```python
from build123d import *

# Parameters (mm, degrees)
BOSS_EXTRUDE1_DEPTH = 6
SKETCH2_W           = 0.8
SKETCH2_H           = 5.9
CUT_EXTRUDE1_DEPTH  = 0.5
SKETCH3_R           = 0.2
BOSS_EXTRUDE2_DEPTH = 2.5


with BuildPart() as part:
    # Sketch1 → Boss-Extrude1 (new body)
    with BuildSketch(Plane(origin=(0, 0, 0), x_dir=(0, 0, -1), z_dir=(1, 0, 0))):
        Polygon((-7.5, -6.8), (-7.5, 3.2), (-2.5, 3.2), (-2.5, -4.8), (2.5, -4.8), (2.5, 3.2), (7.5, 3.2), (7.5, -6.8), align=None)
    extrude(amount=BOSS_EXTRUDE1_DEPTH)

    # Sketch2 → Cut-Extrude1 (cut)
    with BuildSketch(Plane(origin=(0, 0, -7.5), x_dir=(-1, 0, 0), z_dir=(0, 0, -1))):
        with Locations((-3, 0.25)):
            Rectangle(SKETCH2_W, SKETCH2_H)
    cut_extrude1 = extrude(amount=-CUT_EXTRUDE1_DEPTH, mode=Mode.SUBTRACT)

    # Mirror1: Cut-Extrude1 across plane
    add(cut_extrude1.mirror(Plane.XY), mode=Mode.SUBTRACT)

    # Sketch3 → Boss-Extrude2 (add)
    with BuildSketch(Plane.XZ.offset(6.8)):
        with Locations((1.73, -5)):
            Circle(SKETCH3_R)
        with Locations((4.27, -5)):
            Circle(SKETCH3_R)
        with Locations((4.27, 5)):
            Circle(SKETCH3_R)
        with Locations((1.73, 5)):
            Circle(SKETCH3_R)
    extrude(amount=BOSS_EXTRUDE2_DEPTH)


solid = part.part
```
The listing builds one solid part. Answer for the finished solid, in the listing's coordinates (mm). A direction names the side the tool comes from. Round coordinates to 2 decimals unless told otherwise and drop trailing zeros. Loops run counter-clockwise (first coordinate to the right, second up) from the corner with the lowest first, then second, coordinate; pieces in that order, holes last.
Q1. Section D-D, the plane x = 1.73 is taken. Determine the outline of the cut face in (y, z).
Q2. Which of the six approach directions +Z, -Z, +X, -X, +Y, -Y give full straight-line access (tool end or side, diameter ignored) to faces 1 (the face through (3, 3.2, -5)), 2 (the face through (3, -1, 2.5))?
Q3. Section A-A, the plane y = -2 is taken. Determine the outline of the cut face in (x, z).
Q4. Section B-B, the plane x = 5 is taken. Determine the outline of the cut face in (y, z), then the cut area to 3 significant figures.
Q5. Find the intervals of material crossed by line 1 (Z direction, x = 2.65, y = -0.75); line 2 (Z direction, x = 1.6, y = 0.25); line 3 (Y direction, x = 1.05, z = 3.75), in increasing order.
Q6. Section C-C, the plane z = 5 is taken. Determine the outline of the cut face in (x, y).
Q7. Given pin 1 Ø3 at (x, z) = (4, -2.5) entering from -Y; pin 2 Ø3 at (x, y) = (3, 0.5) entering from +Z; pin 3 Ø1.5 at (x, z) = (2, 1) entering from +Y, each flat-ended and moving along its own axis, determine where each tip first touches the part or whether it passes through.
Q8. For a pull along Z with two mould halves and no side action, classify faces 3 (the face through (3, -1, -2.5)), 4 (the face through (3, 3.2, 5)), 5 (the face through (2, -2, 7.5)), 6 (the face through (3, -4.8, 0)) as released by +Z, released by -Z, zero draft, split by the parting line, or undercut.
Completed:
1. outline: (-9.3, -5.2) - (-6.8, -5.2) - (-6.8, -7.5) - (3.2, -7.5) - (3.2, -2.5) - (-4.8, -2.5) - (-4.8, 2.5) - (3.2, 2.5) - (3.2, 7.5) - (-6.8, 7.5) - (-6.8, 5.2) - (-9.3, 5.2) - (-9.3, 4.8) - (-6.8, 4.8) - (-6.8, -4.8) - (-9.3, -4.8) - close
2. face 1: +Z, -Z, +X, -X, +Y
2. face 2: +X, -X, +Y
3. outline: (0, -7.5) - (2.6, -7.5) - (2.6, -7) - (3.4, -7) - (3.4, -7.5) - (6, -7.5) - (6, -2.5) - (0, -2.5) - close; (0, 2.5) - (6, 2.5) - (6, 7.5) - (3.4, 7.5) - (3.4, 7) - (2.6, 7) - (2.6, 7.5) - (0, 7.5) - close
4. outline: (-6.8, -7.5) - (3.2, -7.5) - (3.2, -2.5) - (-4.8, -2.5) - (-4.8, 2.5) - (3.2, 2.5) - (3.2, 7.5) - (-6.8, 7.5) - close
4. area: 110 mm2
5. line 1: z = -7 to -2.5, 2.5 to 7
5. line 2: z = -7.5 to -2.5, 2.5 to 7.5
5. line 3: y = -6.8 to 3.2
6. outline: (0, -6.8) - (1.53, -6.8) - (1.53, -9.3) - (1.93, -9.3) - (1.93, -6.8) - (4.07, -6.8) - (4.07, -9.3) - (4.47, -9.3) - (4.47, -6.8) - (6, -6.8) - (6, 3.2) - (0, 3.2) - close
7. pin 1: stops at y = -6.8
7. pin 2: stops at z = 7.5
7. pin 3: stops at y = -4.8
8. face 3: undercut
8. face 4: zero draft
8. face 5: released by +Z
8. face 6: undercut
